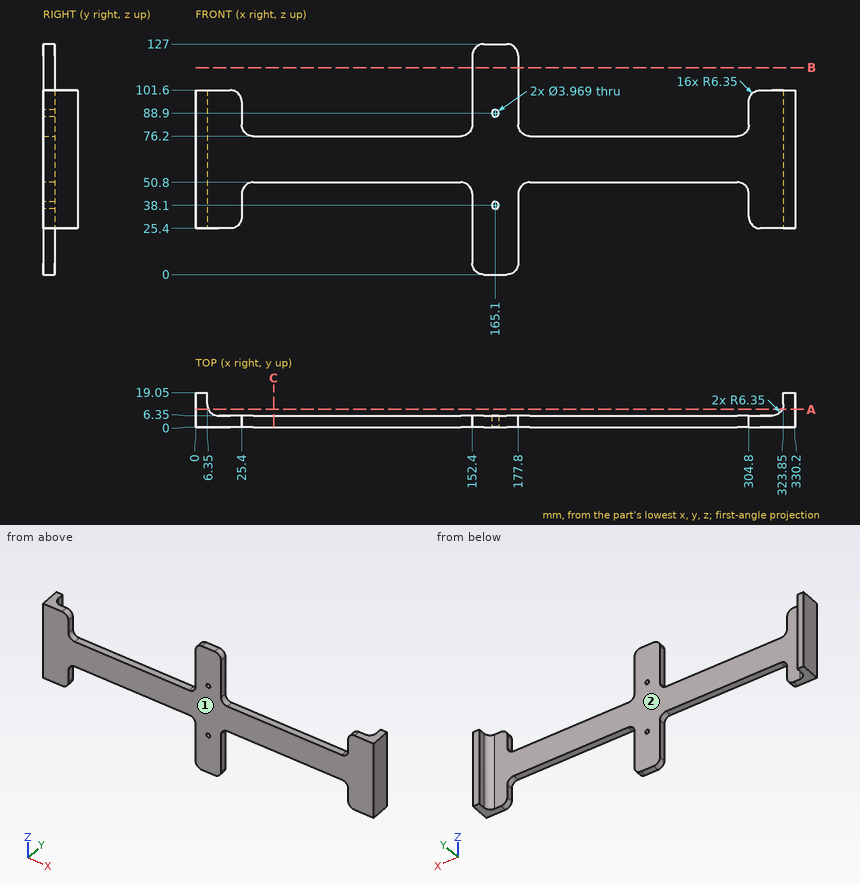
For this review, use the dimensioned drawing (mm, ordinates from the lowest corner) and the shaded views. Round coordinates to 2 decimals unless told otherwise and drop trailing zeros. Order: outer loops, then holes, each group sorted by start corner. A loop starts at its lowest first (then second) coordinate and runs counter-clockwise, first axis right, second up. Notation, with made-up numbers: M -17,7.25 L 22,7.25 A31 ccw 22,45.25 Z; hole C 12,-3.75 d4. An arc over 180 degrees is marked long. Write each question's results on one line, items separated by ' | '. Start each with the question number.
1. Add section C-C (x = 43). State the section outline as (y, z) points.
2. Add section A-A (y = 9.75). State the section outline as (x, z) points.
3. Clearance check with flat-ended pins moving along their axes: pin 1 Ø5.5 at (x, y) = (7, 6) entering from -Z; pin 2 Ø2 at (x, y) = (158, 7.5) entering from -Z; pin 3 Ø1.9 at (y, z) = (4, 109) entering from -X; pin 4 Ø7 at (x, y) = (225, 1.5) entering from -Z. State where each tip first meets the part, or that it passes through.
4. Draft analysis for pull direction X (two halves, no side actions). For the marked faces 1 and 2, state which applies: pulls with the +X half, pulls with the -X half, needs draft (parallel to the pull), parting line crosses it, or undercut.
5. To check wall thickness, follow L1, parallel to Z at x = 165.1, y = 4.25; L2, parallel to X at y = 4, z = 88.9; L3, parallel to X at y = 12, z = 90.5. State the ranges of each line that lie inside material, in increasing order. Write a range as [from, to].
6. Add section B-B (z = 114). State the section outline as (x, y) points.
Output values:
1) outline: M 0,50.8 L 6.35,50.8 L 6.35,76.2 L 0,76.2 Z
2) outline: M 0,25.4 L 7.08,25.4 L 7.08,101.6 L 0,101.6 Z; M 323.12,25.4 L 330.2,25.4 L 330.2,101.6 L 323.12,101.6 Z
3) pin 1: z = 25.4 | pin 2: through | pin 3: x = 152.4 | pin 4: z = 50.8
4) face 1: needs draft | face 2: undercut
5) L1: [0, 36.12], [40.08, 86.92], [90.88, 127] | L2: [0, 25.4], [152.4, 163.12], [167.08, 177.8], [304.8, 330.2] | L3: [0, 6.39], [323.81, 330.2]
6) outline: M 152.4,0 L 177.8,0 L 177.8,6.35 L 152.4,6.35 Z
